from build123d import *

# Parameters (mm, degrees)
F0_W      = 100
F0_H      = 40
F1_DEPTH  = 10
F3_R      = 5
F4_R      = 5
F5_R      = 5
F6_R      = 5
F7_DEPTH  = 25
F8_T      = -2.5
F9_R      = 5
F10_R     = 5
F12_D     = 5
F13_W     = 40
F13_H     = 3
F14_DEPTH = 40.001


# Not quite as in the source:
# - a shell that OpenCascade refuses in one call is made with other operations: the cavity is built on its own and cut out


with BuildPart() as f1:
    # F0 (on Top) → F1 (new body)
    with BuildSketch(Plane.XY):
        with Locations((50, -20)):
            Rectangle(F0_W, F0_H)
    extrude(amount=F1_DEPTH)

    # F3
    f3_edges = [f1.edges().sort_by_distance(p)[0] for p in [
        (100, -40, 5),
    ]]
    fillet(f3_edges, radius=F3_R)

    # F4
    f4_edges = [f1.edges().sort_by_distance(p)[0] for p in [
        (100, 0, 5),
    ]]
    fillet(f4_edges, radius=F4_R)

    # F5
    f5_edges = [f1.edges().sort_by_distance(p)[0] for p in [
        (0, -40, 5),
    ]]
    fillet(f5_edges, radius=F5_R)

    # F6
    f6_edges = [f1.edges().sort_by_distance(p)[0] for p in [
        (0, 0, 5),
    ]]
    fillet(f6_edges, radius=F6_R)

    # F2 (on face) → F7 (join)
    with BuildSketch(Plane.XZ.offset(40)):
        with BuildLine():
            Line((30, 35), (30, 10))
            Line((30, 10), (70, 10))
            Line((70, 10), (70, 35))
            ThreePointArc((70, 35), (50, 55), (30, 35))
        make_face()
    extrude(amount=-F7_DEPTH)

    # F8: a shell. OpenCascade refuses it in one call, so the cavity is built on its own and cut out:
    # the body offset inwards by the wall thickness, plus a prism from it out through each open face.
    f8_core = offset(f1.part, amount=F8_T, kind=Kind.INTERSECTION, mode=Mode.PRIVATE)
    f8_exits = [f8_core.faces().sort_by_distance(p)[0] for p in [
        (50, -2.5, 5),
    ]]
    add(f8_core, mode=Mode.SUBTRACT)
    extrude(f8_exits, amount=-F8_T, mode=Mode.SUBTRACT)

    # F9
    f9_edges = [f1.edges().sort_by_distance(p)[0] for p in [
        (30, -40, 22.5),
    ]]
    fillet(f9_edges, radius=F9_R)

    # F10
    f10_edges = [f1.edges().sort_by_distance(p)[0] for p in [
        (30, -15, 22.5),
    ]]
    fillet(f10_edges, radius=F10_R)

    # F12 (through all)
    with Locations(Plane.XZ.offset(40)):
        with Locations((50, 35)):
            Hole(F12_D / 2)

    # F13 (on face) → F14 (cut, through all)
    with BuildSketch(Plane.XZ.offset(40)):
        with Locations((50, 1.5)):
            Rectangle(F13_W, F13_H)
    extrude(amount=-F14_DEPTH, mode=Mode.SUBTRACT)


solid = f1.part
Could you check a few things on this model? Use its own coordinates, in mm. A direction names the side the tool comes from. Round coordinates to 2 decimals unless told otherwise and drop trailing zeros. Order: outer loops, then holes, each group sorted by start corner. A loop starts at its lowest first (then second) coordinate and runs counter-clockwise, first axis right, second up.
Q1. Thinking about a two-plate mould opening in Z: for faces 4 (the face through (50, -28, 55)), 5 (the face through (50, -17.5, 30)), 6 (the face through (47.69, -38.73, 34.04)), which applies, released by +Z, released by -Z, zero draft, split by the parting line, or undercut?
Geometry says:
face 4: released by +Z
face 5: zero draft
face 6: undercut
Q2. I'm going to push flat-ended pins straight in: P1, Ø10, axis at x = 34, z = 20, coming from the +Y side; P2, Ø1.2, axis at x = 49.5, y = -38.5, coming from the -Z side; P3, Ø0.8, axis at y = -1, z = 4.5, coming from the +X side; P4, Ø6, axis at y = -9.5, z = 43, coming from the +X side. Where does each tip first touch, or does it pass through?
Geometry says:
P1: stops at y = -15
P2: stops at z = 3
P3: stops at x = 98.47
P4: passes through
Q3. Imagine slicing it at A-A, the plane x = 50. List the corners of the cut face in (y, z) for me, then the cut area to 3 significant figures.
Geometry says:
outline: (-40, 3) - (-37.5, 3) - (-37.5, 32.5) - (-40, 32.5) - close; (-40, 37.5) - (-37.5, 37.5) - (-37.5, 52.5) - (-17.5, 52.5) - (-17.5, 37.5) - (-15, 37.5) - (-15, 50) arc R5 ccw to (-20, 55) - (-35, 55) arc R5 ccw to (-40, 50) - close; (-17.5, 7.5) - (0, 7.5) - (0, 10) - (-15, 10) - (-15, 32.5) - (-17.5, 32.5) - close
area: 301 mm2
Q4. Please list where these lines run through material, in increasing order: probe 1 along Y at (x, z) = (53.5, 40); probe 2 along Z at (x, y) = (11, -20); probe 3 along X at (y, z) = (-35, 12.5).
Geometry says:
probe 1: y = -40 to -37.5, -17.5 to -15
probe 2: z = 0 to 2.5, 7.5 to 10
probe 3: x = 30 to 32.5, 67.5 to 70
Q5. Imagine slicing it at C-C, the plane x = 18. List the corners of the cut face in (y, z) for me, then the cut area to 4 significant figures.
Geometry says:
outline: (-40, 0) - (0, 0) - (0, 2.5) - (-37.5, 2.5) - (-37.5, 7.5) - (0, 7.5) - (0, 10) - (-40, 10) - close
area: 212.5 mm2
Q6. Imagine slicing it at B-B, the plane z = 22. List the corners of the cut face in (x, y) for me.
Geometry says:
outline: (30, -35) arc R5 ccw to (35, -40) - (65, -40) arc R5 ccw to (70, -35) - (70, -20) arc R5 ccw to (65, -15) - (35, -15) arc R5 ccw to (30, -20) - close; hole (32.5, -37.5) - (67.5, -37.5) - (67.5, -17.5) - (32.5, -17.5) - close
Q7. Imagine slicing it at D-D, the plane y = -8. List the corners of the cut face in (x, z) for me.
Geometry says:
outline: (0, 0) - (30, 0) - (30, 2.5) - (2.5, 2.5) - (2.5, 7.5) - (97.5, 7.5) - (97.5, 2.5) - (70, 2.5) - (70, 0) - (100, 0) - (100, 10) - (0, 10) - close
Q8. Which directions (+Z, -Z, +X, -X, +Y, -Y) give clear straight access to the entire face, cutting with the end or side of a thin tool? Please do faces 1 (the face through (96.748, -36.787, 5.035)), 2 (the face through (5, -1, 5)), 3 (the face through (50.385, -27.64, 52.496)).
Geometry says:
face 1: none
face 2: +Y
face 3: -Z
